The listing builds one solid part. Answer for the finished solid, in the listing's coordinates (mm). Face numbers are marked on the shaded views. A direction names the side the tool comes from. Round coordinates to 2 decimals unless told otherwise and drop trailing zeros. Order: outer loops, then holes, each group sorted by start corner. A loop starts at its lowest first (then second) coordinate and runs counter-clockwise, first axis right, second up. Notation, with made-up numbers: M -4,25.25 L 15,25.25 A20 ccw 15,44.25 Z; hole C 52,23 d7. An arc over 180 degrees is marked long. Put each result on its own line as item: value. Start each with the question number.
1. The part is cut by section B-B (z = 12). Give the vertices of the cut face in (x, y) (3 decimals), then the cut area to 3 significant figures.
2. Consider line 1 (X direction, y = 11.25, z = 12); line 2 (Y direction, x = 5.75, z = 4.75); line 3 (Z direction, x = 4.5, y = -0.25). Determine where each line is inside the solid, lowest interval first.
3. This flat-tipped pin is pushed along its axis until it touches: pin 1 Ø1 at (x, y) = (-0.5, -7.5) entering from +Z. Where does it stop, or does it pass through?
4. The part is cut by section D-D (y = 1.25). Give the vertices of the cut face in (x, z) (3 decimals).
5. The part is cut by section C-C (z = 6.5). Give the vertices of the cut face in (x, y).
6. The part is cut by section A-A (x = 0). Give the vertices of the cut face in (y, z) (3 decimals).
7. The mould has two halves that part along X. Classify the marked faces 1, 2 and 3: +X half, -X half, draft (parallel to the pull), parting line (faces both ways), or undercut.
8. Which of the six approach directions +Z, -Z, +X, -X, +Y, -Y give full straight-line access (tool end or side, diameter ignored) to the marked faces 4 and 5?
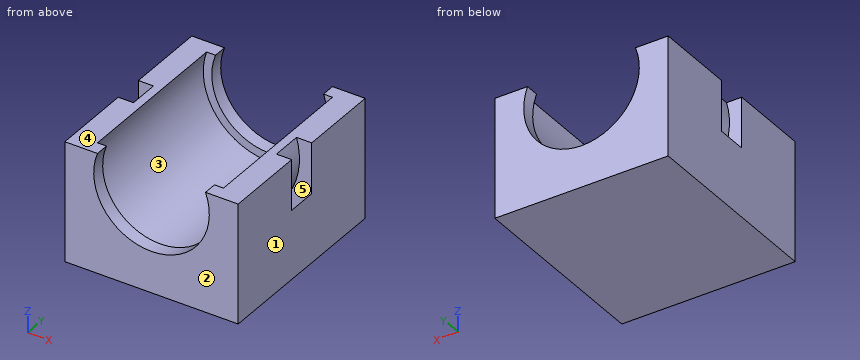
from build123d import *

# Parameters (mm, degrees)
PAD002_DEPTH = 1.85
SKETCH001_R  = 8.025
PAD001_DEPTH = 10.05
SKETCH_W     = 21
SKETCH_H     = 23.4
PAD_DEPTH    = 14.5
SKETCH002_R  = 7
POCKET_DEPTH = 23.401


with BuildPart() as pad002:
    # Sketch003 → Pad002 (new body, symmetric)
    with BuildSketch(Plane.XZ):
        with BuildLine():
            Line((-8.5, 15), (-10.7, 15))
            ThreePointArc((-10.7, 15), (0, 0.887395), (10.7, 15))
            Line((8.5, 15), (10.7, 15))
            ThreePointArc((-8.5, 15), (0, 2.986122), (8.5, 15))
        make_face()
    extrude(amount=PAD002_DEPTH, both=True)


with BuildPart() as pad001:
    # Sketch001 → Pad001 (new body, symmetric)
    with BuildSketch(Plane.XZ):
        with Locations((0, 12)):
            Circle(SKETCH001_R)
    extrude(amount=PAD001_DEPTH, both=True)


with BuildPart() as cut001:
    # Sketch → Pad (new body)
    with BuildSketch(Plane.XY):
        Rectangle(SKETCH_W, SKETCH_H)
    extrude(amount=PAD_DEPTH)

    # Cut: cut Pad001
    add(pad001.part, mode=Mode.SUBTRACT)

    # Sketch002 → Pocket (cut, through all)
    with BuildSketch(Plane.XZ.offset(11.7)):
        with Locations((0, 12)):
            Circle(SKETCH002_R)
    extrude(amount=-POCKET_DEPTH, mode=Mode.SUBTRACT)

    # Cut001: cut Pad002
    add(pad002.part, mode=Mode.SUBTRACT)


solid = cut001.part
Resolved:
1. outline: M -10.5,-11.7 L -7,-11.7 L -7,-10.05 L -8.025,-10.05 L -8.025,10.05 L -7,10.05 L -7,11.7 L -10.5,11.7 L -10.5,1.85 L -9.014,1.85 L -9.014,-1.85 L -10.5,-1.85 Z; M 7,-11.7 L 10.5,-11.7 L 10.5,-1.85 L 9.014,-1.85 L 9.014,1.85 L 10.5,1.85 L 10.5,11.7 L 7,11.7 L 7,10.05 L 8.025,10.05 L 8.025,-10.05 L 7,-10.05 Z
1. area: 112 mm2
2. line 1: -10.5 to -7, 7 to 10.5
2. line 2: -11.7 to -1.85, 1.85 to 11.7
2. line 3: 0 to 1.84, 4.19 to 5.36
3. pin 1: z = 4.04
4. outline: M -10.5,0 L 10.5,0 L 10.5,8.361 A11.113 cw -10.5,8.361 Z; M -8.66,14.5 A9.014 ccw long 8.66,14.5 L 7.626,14.5 A8.025 cw long -7.626,14.5 Z
5. outline: M -10.5,-11.7 L -4.33,-11.7 L -4.33,-10.05 L -5.84,-10.05 L -5.84,10.05 L -4.33,10.05 L -4.33,11.7 L -10.5,11.7 Z; M 4.33,-11.7 L 10.5,-11.7 L 10.5,11.7 L 4.33,11.7 L 4.33,10.05 L 5.84,10.05 L 5.84,-10.05 L 4.33,-10.05 Z; hole M -9.66,-1.85 L -7.14,-1.85 L -7.14,1.85 L -9.66,1.85 Z; hole M 7.14,-1.85 L 9.66,-1.85 L 9.66,1.85 L 7.14,1.85 Z
6. outline: M -11.7,0 L 11.7,0 L 11.7,5 L 10.05,5 L 10.05,3.975 L -10.05,3.975 L -10.05,5 L -11.7,5 Z; hole M -1.85,0.887 L 1.85,0.887 L 1.85,2.986 L -1.85,2.986 Z
7. face 1: +X half
7. face 2: draft
7. face 3: undercut
8. face 4: +Z, +X, -X, +Y, -Y
8. face 5: none
